Geometry check sheet. Reference: the model listing, model coordinates, mm. Face numbers are marked on the shaded views. A direction names the side the tool comes from. Give positions to 0.01 mm unless a question says otherwise; leave off trailing zeros. Loops run counter-clockwise (first coordinate to the right, second up) from the corner with the lowest first, then second, coordinate; pieces in that order, holes last. Notation, with made-up numbers: (72.25, 48) -> (85.25, 48) arc R10 ccw to (85.25, 67) -> close; hole circle Ø1 at (-22.75, 21.25). An arc over 180 degrees is marked (long way). One line per question, with ' | ' between items.
from build123d import *

# Parameters (mm, degrees)
F0_W     = 800
F0_H     = 300
F1_DEPTH = 25
F2_W     = 50
F2_H     = 100
F3_DEPTH = 75
F4_W     = 25
F4_H     = 100
F5_DEPTH = 300
F6_R     = 12.5
F7_DEPTH = 75
F8_W     = 650
F8_H     = 150
F9_DEPTH = 25
F10_R    = 50
F11_R    = 50


with BuildPart() as f1:
    # F0 (on Front) → F1 (new body)
    with BuildSketch(Plane.XZ):
        Rectangle(F0_W, F0_H)
    extrude(amount=F1_DEPTH)

    # F2 (on face) → F3 (join)
    with BuildSketch(Plane(origin=(0, 0, 0), x_dir=(-1, 0, 0), z_dir=(0, 1, 0))):
        with Locations((-375, -100)):
            Rectangle(F2_W, F2_H)
    extrude(amount=F3_DEPTH)

    # F4 (on face) → F5 (join)
    with BuildSketch(Plane.YZ.offset(400)):
        with Locations((62.5, -100)):
            Rectangle(F4_W, F4_H)
    extrude(amount=F5_DEPTH)

    # F6 (on face) → F7 (join)
    with BuildSketch(Plane.XZ.offset(-50)):
        with Locations((635, -78)):
            Circle(F6_R)
    extrude(amount=F7_DEPTH)

    # F8 (on face) → F9 (cut)
    with BuildSketch(Plane.XZ.offset(25)):
        with Locations((-75, -75)):
            Rectangle(F8_W, F8_H)
    extrude(amount=-F9_DEPTH, mode=Mode.SUBTRACT)

    # F10
    f10_edges = [f1.edges().sort_by_distance(p)[0] for p in [
        (-400, -12.5, 0),
        (250, -12.5, 0),
        (250, -12.5, -150),
    ]]
    fillet(f10_edges, radius=F10_R)

    # F11
    f11_edges = [f1.edges().sort_by_distance(p)[0] for p in [
        (-400, -12.5, 150),
    ]]
    fillet(f11_edges, radius=F11_R)


solid = f1.part
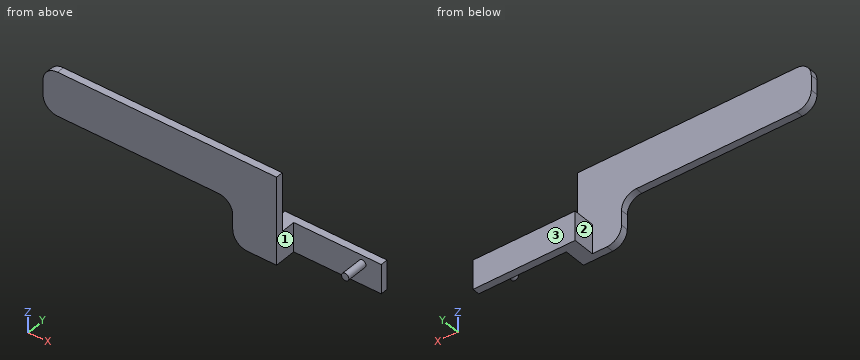
Item 1: Set-up check for the marked faces 1, 2 and 3: record each of +Z, -Z, +X, -X, +Y, -Y from which the full face is reachable in a straight line by a thin tool's end or side.
Result:
face 1: +Z, -Z, -Y | face 2: +Z, -Z, -X, +Y | face 3: +Z, -Z, +X, -X, +Y
Item 2: Sectioned sample at D-D (z = 38). Record the cut outline in (x, y), plus the area to 3 significant figures.
Result:
outline: (-398.54, -25) -> (400, -25) -> (400, 0) -> (-398.54, 0) -> close | area: 20,000 mm2
Item 3: Depth check by flat-ended pin: pin 1 Ø6 at (y, z) = (10, -112) entering from -X; pin 2 Ø22.5 at (x, y) = (603, 45) entering from +Z; pin 3 Ø1 at (y, z) = (-2, -41) entering from -X. Enter the tip coordinate at first touch or a pass-through.
Result:
pin 1: x = 350 | pin 2: z = -50 | pin 3: x = 249.09
Item 4: Sectioned sample at C-C (x = 135). Record the cut outline in (y, z), plus the area to 3 significant figures.
Result:
outline: (-25, 0) -> (0, 0) -> (0, 150) -> (-25, 150) -> close | area: 3,750 mm2
Item 5: Sectioned sample at A-A (x = 635). Record the cut outline in (y, z).
Result:
outline: (-25, -90.5) -> (50, -90.5) -> (50, -150) -> (75, -150) -> (75, -50) -> (50, -50) -> (50, -65.5) -> (-25, -65.5) -> close
Item 6: Scan lines: probe 1 along Y at (x, z) = (245, 73.5); probe 2 along Z at (x, y) = (389, 61); probe 3 along Y at (x, z) = (543, -54). Record each from-to range of solid material in increasing order.
Result:
probe 1: -25 to 0 | probe 2: -150 to -50 | probe 3: 50 to 75
Item 7: Sectioned sample at B-B (z = -78). Record the cut outline in (x, y), plus the area to 3 significant figures.
Result:
outline: (250, -25) -> (400, -25) -> (400, 50) -> (622.5, 50) -> (622.5, -25) -> (647.5, -25) -> (647.5, 50) -> (700, 50) -> (700, 75) -> (350, 75) -> (350, 0) -> (250, 0) -> close | area: 16,900 mm2
